```python
from build123d import *

# Parameters (mm, degrees)
F0_R     = 9.5
F0_R_2   = 7.5
F1_DEPTH = 80
F2_W     = 5
F2_H     = 11
F3_DEPTH = 25
F4_DEPTH = 2


with BuildPart() as f1:
    # F0 (on Top) → F1 (new body)
    with BuildSketch(Plane.XY):
        Circle(F0_R)
        Circle(F0_R_2, mode=Mode.SUBTRACT)
    extrude(amount=F1_DEPTH)

    # F2 (on Right) → F3 (cut)
    with BuildSketch(Plane.YZ):
        with Locations((0, 60)):
            Rectangle(F2_W, F2_H)
    extrude(amount=-F3_DEPTH, mode=Mode.SUBTRACT)

    # F0 (on Top) → F4 (join)
    with BuildSketch(Plane.XY):
        Circle(F0_R_2)
    extrude(amount=F4_DEPTH)


solid = f1.part
```
Check sheet for the modelled part. Datum: model origin and axes. Units: mm. A direction names the side the tool comes from. Coordinates: 2 decimals unless noted, no trailing zeros. Loops run counter-clockwise (first coordinate to the right, second up) from the corner with the lowest first, then second, coordinate; pieces in that order, holes last.
1) Sectioned sample at B-B (x = 0). Record the boundary of the cut face in (y, z), and give its area (3 significant figures).
2) Access from +Z, -Z, +X, -X, +Y, -Y to the whole of each face (thin tool, end or side, straight path). Record for faces 4 (the face through (-8, 0, 65.5)), 5 (the face through (1, 8, 80)), 6 (the face through (0, 0, 2)).
3) Sectioned sample at C-C (z = 48). Record the boundary of the cut face in (x, y).
4) Release check for a two-part mould opening along X. For faces 1 (the face through (7.154, 2.253, 40.454)), 2 (the face through (8.776, -3.639, 39.44)), 3 (the face through (-8, 0, 54.5)) record: released by +X, released by -X, zero draft, split by the parting line, or undercut.
5) Sectioned sample at D-D (y = 5.25). Record the boundary of the cut face in (x, z), and give its area (3 significant figures).
6) Material ranges on probe 1 along Y at (x, z) = (0.5, 29); probe 2 along Z at (x, y) = (-0.25, 5.75); probe 3 along Y at (x, z) = (-5.5, 62), recorded low to high.
7) Gauge pin test, flat ends, axial feed: pin 1 (1.5 mm diameter, centred on x = 6, y = -6.5, fed in from -Z); pin 2 (4.5 mm diameter, centred on x = 3.5, y = 0.5, fed in from +Z); pin 3 (4 mm diameter, centred on y = 3, z = 56, fed in from +X); pin 4 (1 mm diameter, centred on x = -8.5, z = 59.5, fed in from +Y). Record the tip position at first contact, or that the pin passes through.
8) Sectioned sample at A-A (y = 0). Record the boundary of the cut face in (x, z).
Check sheet entries:
1. outline: (-9.5, 0) - (9.5, 0) - (9.5, 80) - (7.5, 80) - (7.5, 2) - (-7.5, 2) - (-7.5, 80) - (-9.5, 80) - close
1. area: 350 mm2
2. face 4: -X
2. face 5: +Z, +X, -X, +Y, -Y
2. face 6: +Z
3. outline: circle Ø19 at (0, 0); hole circle Ø15 at (0, 0)
4. face 1: undercut
4. face 2: split by the parting line
4. face 3: zero draft
5. outline: (-7.92, 0) - (7.92, 0) - (7.92, 80) - (5.36, 80) - (5.36, 2) - (-5.36, 2) - (-5.36, 80) - (-7.92, 80) - close
5. area: 431 mm2
6. probe 1: y = -9.49 to -7.48, 7.48 to 9.49
6. probe 2: z = 0 to 2
6. probe 3: y = -7.75 to -5.1, 5.1 to 7.75
7. pin 1: stops at z = 0
7. pin 2: stops at z = 2
7. pin 3: stops at x = 9.45
7. pin 4: stops at y = 5.12
8. outline: (-9.5, 0) - (9.5, 0) - (9.5, 80) - (7.5, 80) - (7.5, 2) - (-7.5, 2) - (-7.5, 54.5) - (-9.5, 54.5) - close; (-9.5, 65.5) - (-7.5, 65.5) - (-7.5, 80) - (-9.5, 80) - close
